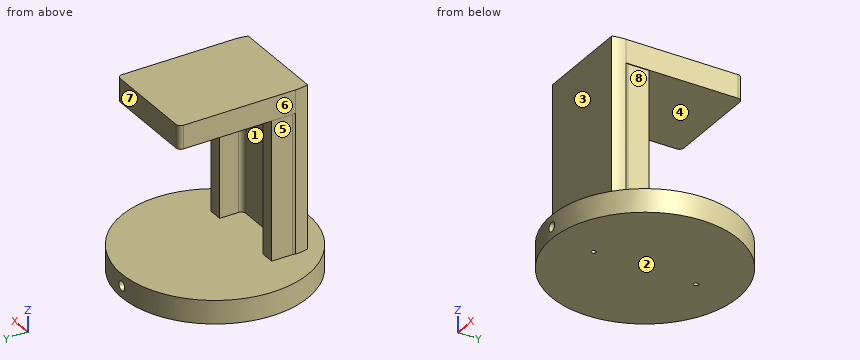
from build123d import *

# Parameters (mm, degrees)
SKETCH1_R               = 20
BOSS_EXTRUDE1_DEPTH     = 5
BOSS_EXTRUDE2_DEPTH     = 34.79
SKETCH3_W               = 21.3
SKETCH3_H               = 5
BOSS_EXTRUDE3_DEPTH     = 25
SKETCH4_W               = 3
SKETCH4_H               = 29.79
BOSS_EXTRUDE5_DEPTH     = 5
CUT_EXTRUDE1_DEPTH      = 38
CUT_EXTRUDE1_DEPTH_BACK = 45.836860952
SKETCH5_R               = 1
FILLET1_R               = 1
FILLET2_R               = 1
FILLET3_R               = 1
CUT_EXTRUDE2_REACH      = 50.818
CUT_EXTRUDE2_END_RADIUS = 1
SKETCH6_R               = 0.5


with BuildPart() as part:
    # Sketch1 → Boss-Extrude1 (new body)
    with BuildSketch(Plane.XY):
        Circle(SKETCH1_R)
    extrude(amount=-BOSS_EXTRUDE1_DEPTH)

    # Sketch2 → Boss-Extrude2 (add)
    with BuildSketch(Plane.XY):
        with BuildLine():
            Line((-10.65, -10.65), (10.65, -10.65))
            ThreePointArc((10.65, -10.65), (10.553147336, -12.083032205), (10.264350929, -13.49))
            Line((10.264350929, -13.49), (-10.264350929, -13.49))
            ThreePointArc((-10.264350929, -13.49), (-10.553147336, -12.083032205), (-10.65, -10.65))
        make_face()
    extrude(amount=BOSS_EXTRUDE2_DEPTH)

    # Sketch3 → Boss-Extrude3 (add)
    with BuildSketch(Plane(origin=(0, -10.65, 0), x_dir=(1, 0, 0), z_dir=(0, 1, 0))):
        with Locations((0, -32.29)):
            Rectangle(SKETCH3_W, SKETCH3_H)
    extrude(amount=BOSS_EXTRUDE3_DEPTH)

    # Sketch4 → Boss-Extrude5 (add)
    with BuildSketch(Plane(origin=(0, -10.65, 0), x_dir=(1, 0, 0), z_dir=(0, 1, 0))):
        with Locations((9, -14.895)):
            Rectangle(SKETCH4_W, SKETCH4_H)
        with Locations((-9, -14.895)):
            Rectangle(SKETCH4_W, SKETCH4_H)
    extrude(amount=BOSS_EXTRUDE5_DEPTH)

    # Sketch5 → Cut-Extrude1 (cut, two sides: drawn at the far end of the back side and taken through both)
    with BuildSketch(Plane(origin=(0, 0, 0), x_dir=(1, 0, 0), z_dir=(0, 1, 0)).offset(-CUT_EXTRUDE1_DEPTH_BACK)):
        with Locations(Location((0, 2.5, 0), (0, 0, 90))):
            Circle(SKETCH5_R)
    extrude(amount=CUT_EXTRUDE1_DEPTH + CUT_EXTRUDE1_DEPTH_BACK, mode=Mode.SUBTRACT)

    # Fillet1
    fillet1_edges = [part.edges().sort_by_distance(p)[0] for p in [
        (10.65, 14.35, 32.29),
        (-10.65, 14.35, 32.29),
    ]]
    fillet(fillet1_edges, radius=FILLET1_R)

    # Fillet2
    fillet2_edges = [part.edges().sort_by_distance(p)[0] for p in [
        (7.5, -10.65, 14.895),
        (-7.5, -10.65, 14.895),
    ]]
    fillet(fillet2_edges, radius=FILLET2_R)

    # Fillet3
    # the kernel refuses this fillet: 1 mm, written as the material it adds along each edge
    with BuildSketch(Plane(origin=(10.5, -10.65, 31.106956719), x_dir=(0, 1, 0), z_dir=(0, 0, -1))) as fillet3_piece_1:
        with BuildLine():
            CenterArc((0.526782688, 1), FILLET3_R, 238.211669382, 31.788330618)
            Line((0, 0.15), (-0.010535654, 0.133))
            ThreePointArc((-0.010535654, 0.133), (-0.02, 0.075), (-0.02, 0))
            Line((-0.02, 0), (0, -0.02))
            Line((0, -0.02), (0.526782688, -0.02))
            Line((0.526782688, -0.02), (0.526782688, 0))
        make_face()
    extrude(amount=32.423913438)
    with BuildSketch(Plane(origin=(-10.5, -10.65, 31.106956719), x_dir=(0, 1, 0), z_dir=(0, 0, -1))) as fillet3_piece_2:
        with BuildLine():
            CenterArc((0.526782688, -1), FILLET3_R, 90, 31.788330618)
            Line((0, -0.15), (-0.010535654, -0.133))
            ThreePointArc((-0.010535654, -0.133), (-0.02, -0.075), (-0.02, 0))
            Line((-0.02, 0), (0, 0.02))
            Line((0, 0.02), (0.526782688, 0.02))
            Line((0.526782688, 0.02), (0.526782688, 0))
        make_face()
    extrude(amount=32.423913438)

    # Cut-Extrude2: up to this cylinder (the profile starts outside it)
    cut_extrude2_end = Plane(origin=(0, 0, -2.5), z_dir=(0, -1, 0)) * Cylinder(CUT_EXTRUDE2_END_RADIUS, 126.636, mode=Mode.PRIVATE)
    # Sketch6 → Cut-Extrude2 (cut, up to the surface)
    with BuildSketch(Plane(origin=(0, 0, -5), x_dir=(-1, 0, 0), z_dir=(0, 0, -1)), mode=Mode.PRIVATE) as cut_extrude2_sk1:
        with Locations((0, 11)):
            Circle(SKETCH6_R)
    cut_extrude2_tool1 = extrude(cut_extrude2_sk1.sketch, amount=-CUT_EXTRUDE2_REACH, mode=Mode.PRIVATE) - cut_extrude2_end
    add(cut_extrude2_tool1.solids().sort_by_distance((0, 11, -5))[0], mode=Mode.SUBTRACT)
    # Sketch6 → Cut-Extrude2 (cut, up to the surface)
    with BuildSketch(Plane(origin=(0, 0, -5), x_dir=(-1, 0, 0), z_dir=(0, 0, -1)), mode=Mode.PRIVATE) as cut_extrude2_sk2:
        with Locations((0, -11)):
            Circle(SKETCH6_R)
    cut_extrude2_tool2 = extrude(cut_extrude2_sk2.sketch, amount=-CUT_EXTRUDE2_REACH, mode=Mode.PRIVATE) - cut_extrude2_end
    add(cut_extrude2_tool2.solids().sort_by_distance((0, -11, -5))[0], mode=Mode.SUBTRACT)


solid = part.part
Input: part model. Units: mm. Frame: model coordinates. Face numbers are marked on the shaded views. A direction names the side the tool comes from. Coordinates: 2 decimals unless noted, no trailing zeros. Loops run counter-clockwise (first coordinate to the right, second up) from the corner with the lowest first, then second, coordinate; pieces in that order, holes last. Notation, with made-up numbers: (33, 50) - (53, 50) arc R10 ccw to (53, 63) - close; hole circle Ø2 at (3.25, -38). An arc over 180 degrees is marked (long way). Answer in a Markdown table with one row per item. Add a question column.
Item 1: Section query A-A on y = 8. Return the cut outline in (x, z).
Item 2: Section query C-C on x = 8.5. Return the cut outline in (y, z).
Item 3: Access query for the marked faces 4, 5, 6, 7 and 8. Directions: +Z, -Z, +X, -X, +Y, -Y. A direction counts if a zero-diameter tool reaches every point of the face in a straight line with its end or side. Return the directions, or none.
Item 4: Section query B-B on z = 3.5. Return the cut outline in (x, y).
Item 5: Line query: line 1 along Y through (x, z) = (0, -4.4); line 2 along Z through (x, y) = (-8, -5); line 3 along Z through (x, y) = (6.5, -14.5). Output: solid intervals per line, ascending. Write a range as [from, to].
Item 6: Contact query for flat-ended pins moving along their axis: P1, Ø1.5, axis at y = -2.5, z = 32, coming from the +X side; P2, Ø1.5, axis at y = -3, z = 33.5, coming from the -X side; P3, Ø3.5, axis at x = -8.5, z = 15.5, coming from the +Y side; P4, Ø1, axis at x = 13, z = 10, coming from the +Y side. Output: stop coordinate, or through.
Item 7: Mould query, pull axis Z, two halves, no side actions, for the marked faces 1, 2 and 3. Classes: released by +Z, released by -Z, zero draft, split by the parting line, or undercut.
Recorded:
| question | item | result |
|---|---|---|
| 1 | outline | (-18.33, -5) - (18.33, -5) - (18.33, 0) - (-18.33, 0) - close; (-10.65, 29.79) - (10.65, 29.79) - (10.65, 34.79) - (-10.65, 34.79) - close; hole circle Ø2 at (0, -2.5) |
| 2 | outline | (-18.1, -5) - (18.1, -5) - (18.1, 0) - (-5.65, 0) - (-5.65, 29.79) - (14.35, 29.79) - (14.35, 34.79) - (-13.49, 34.79) - (-13.49, 0) - (-18.1, 0) - close |
| 3 | face 4 | +Y |
| 3 | face 5 | -X, +Y |
| 3 | face 6 | +Z, -X, +Y, -Y |
| 3 | face 7 | +Z, +X, -X, +Y |
| 3 | face 8 | +X, +Y |
| 4 | outline | (-10.65, -10.65) arc R10.65 ccw to (-10.26, -13.49) - (10.26, -13.49) arc R10.65 ccw to (10.65, -10.65) arc R1 cw to (10.5, -10.12) - (10.5, -5.65) - (7.5, -5.65) - (7.5, -9.65) arc R1 cw to (6.5, -10.65) - (-6.5, -10.65) arc R1 cw to (-7.5, -9.65) - (-7.5, -5.65) - (-10.5, -5.65) - (-10.5, -10.12) arc R1 cw to start |
| 5 | line 1 | [-20, -11.5], [-10.5, 10.5], [11.5, 20] |
| 5 | line 2 | [-5, 0], [29.79, 34.79] |
| 5 | line 3 | [-5, 0] |
| 6 | P1 | x = 10.65 |
| 6 | P2 | x = -10.65 |
| 6 | P3 | y = -5.65 |
| 6 | P4 | through |
| 7 | face 1 | undercut |
| 7 | face 2 | released by -Z |
| 7 | face 3 | zero draft |
